Design review of the part built by this model. Coordinates are the model's own, in mm. A direction names the side the tool comes from. Round coordinates to 2 decimals unless told otherwise and drop trailing zeros. Order: outer loops, then holes, each group sorted by start corner. A loop starts at its lowest first (then second) coordinate and runs counter-clockwise, first axis right, second up. Notation, with made-up numbers: (41.5, -40) - (58.5, -40) arc R26 ccw to (58.5, -24) - close; hole circle Ø3 at (-12.5, 55). An arc over 180 degrees is marked (long way). Write item = value, one per line.
from build123d import *

# Parameters (mm, degrees)
BOSS_EXTRUDE1_DEPTH     = 10
FILLET1_R               = 0.987
CUT_EXTRUDE1_DEPTH      = 106.944642895
CUT_EXTRUDE1_DEPTH_BACK = 106.944642895
CUT_EXTRUDE2_DEPTH      = 108.351140461
CUT_EXTRUDE2_DEPTH_BACK = 108.351140461
SKETCH3_R               = 1.75
CUT_EXTRUDE3_DEPTH      = 106.944642895
CUT_EXTRUDE3_DEPTH_BACK = 106.944642895
FILLET2_R               = 3


with BuildPart() as part:
    # Sketch1 → Boss-Extrude1 (new, symmetric)
    with BuildSketch(Plane(origin=(0, 0, 0), x_dir=(1, 0, 0), z_dir=(0, 1, 0))):
        Polygon((-19.4, 0), (19.4, 0), (19.4, 9.2), (0, 107.797571926), (-19.4, 9.2), align=None)
    extrude(amount=BOSS_EXTRUDE1_DEPTH, both=True)

    # Fillet1
    fillet1_edges = [part.edges().sort_by_distance(p)[0] for p in [
        (0, 0, -107.797571926),
    ]]
    fillet(fillet1_edges, radius=FILLET1_R)

    # Sketch2 → Cut-Extrude1 (cut, two sides: drawn at the far end of the back side and taken through both)
    with BuildSketch(Plane(origin=(0, 0, 0), x_dir=(1, 0, 0), z_dir=(0, 1, 0)).offset(-CUT_EXTRUDE1_DEPTH_BACK)):
        Polygon((-14.919848876, 24.2), (-17.871240013, 9.2), (17.871240013, 9.2), (14.919848876, 24.2), align=None)
        Polygon((-11.771698328, 40.2), (-14.526330057, 26.2), (14.526330057, 26.2), (11.771698328, 40.2), align=None)
        Polygon((-8.623547781, 56.2), (-11.37817951, 42.2), (11.37817951, 42.2), (8.623547781, 56.2), align=None)
        Polygon((-5.475397234, 72.2), (-8.230028963, 58.2), (8.230028963, 58.2), (5.475397234, 72.2), align=None)
        with BuildLine():
            Line((-0.966469566, 95.115944337), (-5.081878416, 74.2))
            Line((-5.081878416, 74.2), (5.081878416, 74.2))
            Line((5.081878416, 74.2), (0.966469566, 95.115944337))
            ThreePointArc((0.966469566, 95.115944337), (0, 95.910782356), (-0.966469566, 95.115944337))
        make_face()
    extrude(amount=CUT_EXTRUDE1_DEPTH + CUT_EXTRUDE1_DEPTH_BACK, mode=Mode.SUBTRACT)

    # Sketch3 → Cut-Extrude2 (cut, two sides: drawn at the far end of the back side and taken through both)
    with BuildSketch(Plane(origin=(0, 10, 0), x_dir=(1, 0, 0), z_dir=(0, 1, 0)).offset(-CUT_EXTRUDE2_DEPTH_BACK)):
        with Locations(Location((-12.9, 4.6, 0), (0, 0, 270))):
            Circle(SKETCH3_R)
        with Locations(Location((2.1, 4.6, 0), (0, 0, 270))):
            Circle(SKETCH3_R)
    extrude(amount=CUT_EXTRUDE2_DEPTH + CUT_EXTRUDE2_DEPTH_BACK, mode=Mode.SUBTRACT)

    # Sketch4 → Cut-Extrude3 (cut, two sides: drawn at the far end of the back side and taken through both)
    with BuildSketch(Plane(origin=(0, 0, 0), x_dir=(1, 0, 0), z_dir=(0, 1, 0)).offset(-CUT_EXTRUDE3_DEPTH_BACK)):
        Polygon((14.919848876, 24.2), (14.80179323, 24.8), (12.30179323, 24.8), (11.70179323, 24.2), align=None)
        Polygon((14.644385703, 25.6), (14.526330057, 26.2), (11.70179323, 26.2), (12.30179323, 25.6), align=None)
        Polygon((-12.30179323, 25.6), (-11.70179323, 26.2), (-14.526330057, 26.2), (-14.644385703, 25.6), align=None)
        Polygon((-12.30179323, 24.8), (-14.80179323, 24.8), (-14.919848876, 24.2), (-11.70179323, 24.2), align=None)
        Polygon((-11.37817951, 42.2), (-11.496235156, 41.6), (-9.153642683, 41.6), (-8.553642683, 42.2), align=None)
        Polygon((-11.771698328, 40.2), (-8.553642683, 40.2), (-9.153642683, 40.8), (-11.653642683, 40.8), align=None)
        Polygon((8.553642683, 40.2), (11.771698328, 40.2), (11.653642683, 40.8), (9.153642683, 40.8), align=None)
        Polygon((9.153642683, 41.6), (11.496235156, 41.6), (11.37817951, 42.2), (8.553642683, 42.2), align=None)
        Polygon((5.405492136, 56.2), (8.623547781, 56.2), (8.505492136, 56.8), (6.005492136, 56.8), align=None)
        Polygon((6.005492136, 57.6), (8.348084609, 57.6), (8.230028963, 58.2), (5.405492136, 58.2), align=None)
        Polygon((-8.230028963, 58.2), (-8.348084609, 57.6), (-6.005492136, 57.6), (-5.405492136, 58.2), align=None)
        Polygon((-8.623547781, 56.2), (-5.405492136, 56.2), (-6.005492136, 56.8), (-8.505492136, 56.8), align=None)
        Polygon((2.257341589, 72.2), (5.475397234, 72.2), (5.357341589, 72.8), (2.857341589, 72.8), align=None)
        Polygon((2.857341589, 73.6), (5.199934061, 73.6), (5.081878416, 74.2), (2.257341589, 74.2), align=None)
        Polygon((-5.081878416, 74.2), (-5.199934061, 73.6), (-2.857341589, 73.6), (-2.257341589, 74.2), align=None)
        Polygon((-5.475397234, 72.2), (-2.257341589, 72.2), (-2.857341589, 72.8), (-5.357341589, 72.8), align=None)
    extrude(amount=CUT_EXTRUDE3_DEPTH + CUT_EXTRUDE3_DEPTH_BACK, mode=Mode.SUBTRACT)

    # Fillet2
    fillet2_edges = [part.edges().sort_by_distance(p)[0] for p in [
        (17.871240013, 0, -9.2),
        (-17.871240013, 0, -9.2),
    ]]
    fillet(fillet2_edges, radius=FILLET2_R)


solid = part.part
1) To check wall thickness, follow L1, parallel to X at y = -0.75, z = -4.6; L2, parallel to X at y = -4, z = -29; L3, parallel to X at y = -0.5, z = -23.5. State the ranges of each line that lie inside material, in increasing order. Write a range as from..to.
Findings:
L1 = -19.4..-14.65, -11.15..0.35, 3.85..19.4
L2 = -15.5..-13.98, 13.98..15.5
L3 = -16.59..-15.06, 15.06..16.59
2) We need section C-C on y = -1. Give the number of separate pieces and of enclosed holes in the cut face, and give its area (3 significant figures).
Findings:
separate_pieces = 1
enclosed_holes = 7
area = 767 mm^2
3) For faces 1 (the flat face through (1, 10, -25)), 2 (the flat face through (0, 0, -24.2)), list the 3-axis set-ups (+Z, -Z, +X, -X, +Y, -Y) from which the entire face can be reached by the end or side of a thin tool; tool diameter is ignored.
Findings:
face_1 = +Z, -Z, +X, -X, +Y
face_2 = +Y, -Y
4) Clearance check with flat-ended pins moving along their axes: pin 1 Ø3 at (x, z) = (-11.5, -59) entering from +Y; pin 2 Ø2 at (x, y) = (-4.5, -2.5) entering from +Z; pin 3 Ø1 at (y, z) = (1.5, -76.5) entering from +X; pin 4 Ø1.5 at (y, z) = (-0.5, -71.5) entering from -X. State where each tip first meets the part, or that it passes through.
Findings:
pin_1 = through
pin_2 = 0
pin_3 = 6.26
pin_4 = -7.29
5) We need section A-A on z = -4.6. Write out the cut boundary in (x, y).
Findings:
outline = (-19.4, -10) - (-14.65, -10) - (-14.65, 10) - (-19.4, 10) - close; (-11.15, -10) - (0.35, -10) - (0.35, 10) - (-11.15, 10) - close; (3.85, -10) - (19.4, -10) - (19.4, 10) - (3.85, 10) - close
6) We need section B-B on z = -27.5. Write out the cut boundary in (x, y), and give its area (3 significant figures).
Findings:
outline = (-15.8, -10) - (-14.27, -10) - (-14.27, 10) - (-15.8, 10) - close; (14.27, -10) - (15.8, -10) - (15.8, 10) - (14.27, 10) - close
area = 61.2 mm^2
7) The part is to be moulded in two halves that separate along X. For faces 3 (the cylindrical face through (0.02, -0.14, -95.91)), 4 (the flat face through (-19.4, 0, -5)), 5 (the cylindrical face through (-0.02, -0.14, -103.67)), 6 (the flat face through (19.4, 0, -5)), say which applies: released by +X, released by -X, zero draft, split by the parting line, or undercut.
Findings:
face_3 = undercut
face_4 = released by -X
face_5 = split by the parting line
face_6 = released by +X
